Can you work these out from the model? Positions are in its coordinate system, mm. Face numbers are marked on the shaded views. A direction names the side the tool comes from. Round coordinates to 2 decimals unless told otherwise and drop trailing zeros. Write each loop counter-clockwise with the first axis right and the second up, starting at its lowest first coordinate (ties: lowest second). Pieces come first, ordered by that corner, then holes. Notation, with made-up numbers: (3.25, -3) -> (62.25, -3) arc R8 cw to (62.25, 11) -> close; hole circle Ø10 at (26, 29). An arc over 180 degrees is marked (long way). Write item = value, one per line. Start each with the question number.
1) Imagine slicing it at C-C, the plane z = 11.5. Please give me the cut outline in (x, y).
2) I'm going to push flat-ended pins straight in: pin 1 (1.8 mm diameter, centred on x = 0.5, y = -2, fed in from +Z); pin 2 (3 mm diameter, centred on x = 1, y = -2.5, fed in from -Z) (3 decimals); pin 3 (3 mm diameter, centred on y = -2.5, z = 10, fed in from -X). Where does each tip first touch, or does it pass through?
3) Imagine slicing it at D-D, the plane x = -5. Please give me the cut outline in (y, z) (3 decimals).
4) Thinking about a two-plate mould opening in Z: for the marked faces 1, 2 and 3, which applies, +Z half, -Z half, draft (parallel to the pull), parting line (faces both ways), or undercut?
5) If I drill on line 1 (Z direction, x = 5.5, y = -2.75) (3 decimals); line 2 (Y direction, x = -1.5, z = -9); line 3 (Z direction, x = 1.5, y = -2.5), over which ranges is the centre line in solid material (lowest first)?
6) For the marked faces 4, 5, 6 and 7, which set-ups out of +Z, -Z, +X, -X, +Y, -Y let a thin tool reach every point of the face, with its end or its side?
7) Imagine slicing it at A-A, the plane y = -2.75. Please give me the cut outline in (x, z) (3 decimals).
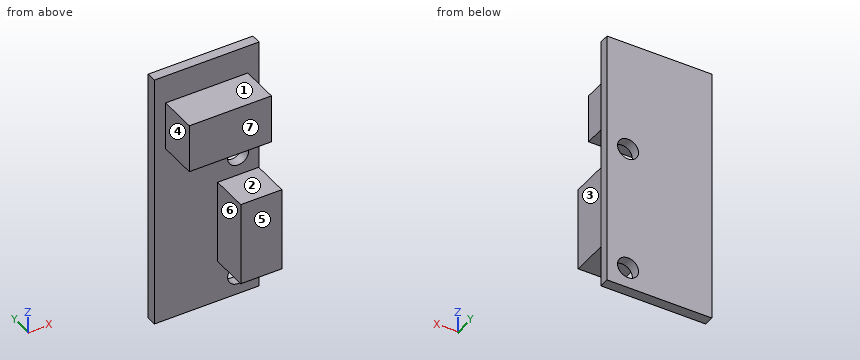
from build123d import *

# Parameters (mm, degrees)
SKETCH1_W           = 15.875
SKETCH1_H           = 39.1414
SKETCH1_R           = 1.5875
SKETCH1_W_2         = 6.223
SKETCH1_H_2         = 12.7
BOSS_EXTRUDE1_DEPTH = 1.524
SKETCH1_4_W         = 3.1115
SKETCH1_4_H         = 12.7
BOSS_EXTRUDE2_DEPTH = 1.524
SKETCH1_5_W         = 3.1115
SKETCH1_5_H         = 12.7
BOSS_EXTRUDE3_DEPTH = 5.715
SKETCH2_W           = 6.223
SKETCH2_H           = 7.366
BOSS_EXTRUDE4_DEPTH = 5.842


with BuildPart() as part:
    # Sketch1 → Boss-Extrude1 (new body)
    with BuildSketch(Plane(origin=(0, 0, 0), x_dir=(1, 0, 0), z_dir=(0, 1, 0))):
        with Locations((0, 2.6543)):
            Rectangle(SKETCH1_W, SKETCH1_H)
        with Locations((4.7625, 19.05)):
            Circle(SKETCH1_R, mode=Mode.SUBTRACT)
        with Locations((4.7625, 0)):
            Circle(SKETCH1_R, mode=Mode.SUBTRACT)
        with Locations((4.7625, 9.525)):
            Rectangle(SKETCH1_W_2, SKETCH1_H_2, mode=Mode.SUBTRACT)
    extrude(amount=BOSS_EXTRUDE1_DEPTH)

    # Sketch1_4 → Boss-Extrude2 (add)
    with BuildSketch(Plane(origin=(0, 0, 0), x_dir=(1, 0, 0), z_dir=(0, 1, 0))):
        with Locations((3.20675, 9.525)):
            Rectangle(SKETCH1_4_W, SKETCH1_4_H)
        with Locations((6.31825, 9.525)):
            Rectangle(SKETCH1_4_W, SKETCH1_4_H)
    extrude(amount=BOSS_EXTRUDE2_DEPTH)

    # Sketch1_5 → Boss-Extrude3 (add)
    with BuildSketch(Plane(origin=(0, 0, 0), x_dir=(1, 0, 0), z_dir=(0, 1, 0))):
        with Locations((6.31825, 9.525)):
            Rectangle(SKETCH1_5_W, SKETCH1_5_H)
        with Locations((3.20675, 9.525)):
            Rectangle(SKETCH1_5_W, SKETCH1_5_H)
    extrude(amount=-BOSS_EXTRUDE3_DEPTH)

    # Sketch2 → Boss-Extrude4 (add)
    with BuildSketch(Plane.XZ):
        with Locations((3.1115, 8.9154)):
            Rectangle(SKETCH2_W, SKETCH2_H)
        with Locations((-3.1115, 8.9154)):
            Rectangle(SKETCH2_W, SKETCH2_H)
    extrude(amount=BOSS_EXTRUDE4_DEPTH)


solid = part.part
Reported:
q1.outline = (-7.94, 0) -> (-6.22, 0) -> (-6.22, -5.84) -> (6.22, -5.84) -> (6.22, 0) -> (7.94, 0) -> (7.94, 1.52) -> (-7.94, 1.52) -> close
q2.pin_1 = 12.6
q2.pin_2 = -15.875
q2.pin_3 = -6.22
q3.outline = (-5.842, 5.232) -> (0, 5.232) -> (0, -22.225) -> (1.524, -22.225) -> (1.524, 16.916) -> (0, 16.916) -> (0, 12.598) -> (-5.842, 12.598) -> close
q4.face_1 = +Z half
q4.face_2 = undercut
q4.face_3 = draft
q5.line_1 = -15.875 to -3.175, 5.232 to 12.598
q5.line_2 = 0 to 1.52
q5.line_3 = 5.23 to 12.6
q6.face_4 = +Z, -Z, -X, -Y
q6.face_5 = -Z, +X, -X, -Y
q6.face_6 = -Z, -X, -Y
q6.face_7 = +Z, -Z, +X, -X, -Y
q7.outline = (-6.223, 5.232) -> (6.223, 5.232) -> (6.223, 12.598) -> (-6.223, 12.598) -> close; (1.651, -15.875) -> (7.874, -15.875) -> (7.874, -3.175) -> (1.651, -3.175) -> close
